Could you check a few things on this model? Use its own coordinates, in mm. A direction names the side the tool comes from. Round coordinates to 2 decimals unless told otherwise and drop trailing zeros. Answer in a Markdown table with one row per item.
```python
from build123d import *

# Parameters (mm, degrees)
F0_R     = 14.20941
F1_DEPTH = 25.4
F2_SIZE  = 2.54
F3_R     = 5.08


with BuildPart() as f1:
    # F0 (on Front) → F1 (new body)
    with BuildSketch(Plane.XZ):
        with BuildLine():
            ThreePointArc((9.975388, -36.042502), (29.762598, -22.644161), (37.397464, 0))
            ThreePointArc((37.397464, 0), (29.783212, 22.617041), (10.041033, 36.024269))
            ThreePointArc((10.041033, 36.024269), (-37.397448, 0.034065), (9.975388, -36.042502))
        make_face()
        Circle(F0_R, mode=Mode.SUBTRACT)
        with BuildLine():
            ThreePointArc((10.041033, 36.024269), (29.783212, 22.617041), (37.397464, 0))
            ThreePointArc((37.397464, 0), (29.762598, -22.644161), (9.975388, -36.042502))
            Line((9.975388, -36.042502), (77.196848, -17.437796))
            ThreePointArc((77.196848, -17.437796), (54.30811, -1.055577), (75.132796, 17.881262))
            Line((75.132796, 17.881262), (10.041033, 36.024269))
        make_face()
        with BuildLine():
            ThreePointArc((90.463979, 0), (86.106461, 11.776934), (75.132796, 17.881262))
            ThreePointArc((75.132796, 17.881262), (54.30811, -1.055577), (77.196848, -17.437796))
            ThreePointArc((77.196848, -17.437796), (86.770139, -10.955518), (90.463979, 0))
        make_face()
        Polygon((66.091331, 5.316778), (67.486724, 6.621571), (69.14541, 7.569393), (70.977968, 8.109147), (72.885606, 8.211735), (74.765481, 7.871627), (76.51625, 7.107156), (78.043527, 5.959538), (79.264978, 4.490639), (80.114752, 2.779648), (80.54704, 0.918806), (80.538535, -0.991569), (80.089696, -2.848488), (79.224722, -4.551845), (77.990241, -6.00981), (76.452806, -7.143785), (74.695301, -7.892637), (72.812471, -8.215995), (70.905823, -8.096426), (69.078143, -7.540377), (67.427962, -6.577824), (66.044242, -5.260659), (65.001579, -3.65989), (64.356184, -1.861816), (64.14285, 0.036629), (64.373079, 1.9331), (65.034457, 3.725356), align=None, mode=Mode.SUBTRACT)
    extrude(amount=F1_DEPTH)

    # F2
    f2_edges = [f1.edges().sort_by_distance(p)[0] for p in [
        (-14.20941, -25.4, 0),
        (75.640865, -25.4, 7.489391),
        (78.607481, -25.4, -5.280828),
        (65.52291, -25.4, -4.460275),
        (77.279888, -25.4, 6.533347),
        (77.221524, -25.4, -6.576798),
        (64.678881, -25.4, -2.760853),
        (78.654252, -25.4, 5.225088),
        (75.574053, -25.4, -7.518211),
        (64.249517, -25.4, -0.912594),
        (79.689865, -25.4, 3.635143),
        (73.753886, -25.4, -8.054316),
        (64.257964, -25.4, 0.984864),
        (68.316067, -25.4, 7.095482),
        (80.330896, -25.4, 1.849227),
        (71.859147, -25.4, -8.15621),
        (64.703768, -25.4, 2.829228),
        (70.061689, -25.4, 7.83927),
        (80.542787, -25.4, -0.036381),
        (69.991983, -25.4, -7.818401),
        (65.562894, -25.4, 4.521067),
        (71.931787, -25.4, 8.160441),
        (80.314116, -25.4, -1.920029),
        (68.253052, -25.4, -7.0591),
        (66.789027, -25.4, 5.969174),
        (73.825543, -25.4, 8.041681),
        (66.736102, -25.4, -5.919241),
        (79.657209, -25.4, -3.700167),
    ]]
    chamfer(f2_edges, length=F2_SIZE)

    # F3
    f3_edges = [f1.edges().sort_by_distance(p)[0] for p in [
        (-16.74941, -25.4, 0),
        (-37.397448, -25.4, 0.034065),
        (43.586118, -25.4, -26.740149),
        (90.433161, -25.4, 1.055577),
        (42.586915, -25.4, 26.952766),
        (76.657281, -25.4, 9.817159),
        (74.277741, -25.4, 10.541104),
        (78.805726, -25.4, 8.563967),
        (71.795389, -25.4, 10.696776),
        (80.607254, -25.4, 6.84909),
        (69.344048, -25.4, 10.275782),
        (81.964744, -25.4, 4.764977),
        (67.055872, -25.4, 9.300818),
        (82.805013, -25.4, 2.423983),
        (65.054216, -25.4, 7.824445),
        (83.082762, -25.4, -0.047689),
        (63.44699, -25.4, 5.926253),
        (82.783017, -25.4, -2.51679),
        (62.32084, -25.4, 3.708576),
        (81.921939, -25.4, -4.85021),
        (61.736477, -25.4, 1.290969),
        (80.545947, -25.4, -6.922154),
        (61.725404, -25.4, -1.196235),
        (78.729221, -25.4, -8.620923),
        (62.288218, -25.4, -3.61895),
        (76.569703, -25.4, -9.854936),
        (63.394579, -25.4, -5.846566),
        (74.183812, -25.4, -10.557666),
        (64.98484, -25.4, -7.758992),
        (71.700172, -25.4, -10.691231),
        (66.973272, -25.4, -9.253129),
        (69.252677, -25.4, -10.248428),
        (43.586118, 0, -26.740149),
    ]]
    fillet(f3_edges, radius=F3_R)


solid = f1.part
```
1) If we mould it in two halves opening along Z, with no side actions, what happens to faces 1 (the face through (43.6, -24, -25.1)), 2 (the face through (61.538, -25.024, -1.196)), 3 (the face through (41.876, -1.449, 25.565))? For each: released by +Z, released by -Z, zero draft, split by the parting line, or undercut.
Computed:
| item | result |
|---|---|
| face 1 | released by -Z |
| face 2 | undercut |
| face 3 | released by +Z |
2) Will these pins go through, and if not, where does the flat tip stop? P1, Ø17, axis at x = 0, z = 0, coming from the -Y side; P2, Ø6, axis at x = 51, y = -14, coming from the -Z side; P3, Ø3, axis at x = -11.5, y = -18, coming from the -Z side; P4, Ø5, axis at y = -18, z = -5, coming from the -X side.
Computed:
| item | result |
|---|---|
| P1 | passes through |
| P2 | stops at z = -25.52 |
| P3 | stops at z = -36.04 |
| P4 | stops at x = -37.31 |
3) I want a section at A-A, the plane y = -6.75. State how many separate pieces and enclosed holes the cut face has, plus the area to 3 significant figures.
Computed:
| item | result |
|---|---|
| separate pieces | 1 |
| enclosed holes | 2 |
| area | 6,020 mm² |
4) I need wall thicknesses on line 1 (Z direction, x = 0, y = -11); line 2 (Z direction, x = 72, y = -8); line 3 (X direction, y = -9, z = -2). Which ranges of each line are inside material? Lowest first, please.
Computed:
| item | result |
|---|---|
| line 1 | z = -37.4 to -14.21, 14.21 to 37.4 |
| line 2 | z = -18.88 to -8.17, 8.16 to 18.75 |
| line 3 | x = -37.34 to -14.07, 14.07 to 64.41, 80.29 to 90.35 |
5) Which directions (+Z, -Z, +X, -X, +Y, -Y) give clear straight access to the entire face, cutting with the end or side of a thin tool? Please do faces 4 (the face through (43.6, -1.4, -25.1)), 5 (the face through (69.178, -25.024, -10.42)).
Computed:
| item | result |
|---|---|
| face 4 | -Z, +X, +Y |
| face 5 | -Y |
